from build123d import *

# Parameters (mm, degrees)
SALIENTE_EXTRUIR1_DEPTH = 3


with BuildPart() as part:
    # Croquis1 → Saliente-Extruir1 (new body)
    with BuildSketch(Plane.XY):
        with BuildLine():
            Line((77.13407836, 15), (-77.13407836, 15))
            add(Edge.make_bspline(
                [(-77.13407836, 15), (-77.871262638, 15), (-78.576496818, 14.787307583), (-79.282235227, 14.574463094), (-79.896125243, 14.167315569)],
                knots=[0, 0, 0, 0.5, 0.5, 1, 1, 1], degree=2))
            ThreePointArc((-79.896125243, 14.167315569), (-87.5, 0), (-79.896125243, -14.167315569))
            add(Edge.make_bspline(
                [(-79.896125243, -14.167315569), (-79.281776873, -14.574767086), (-78.576496886, -14.787307562), (-77.870712638, -15), (-77.13407836, -15)],
                knots=[0, 0, 0, 0.5, 0.5, 1, 1, 1], degree=2))
            Line((-77.13407836, -15), (77.13407836, -15))
            add(Edge.make_bspline(
                [(77.13407836, -15), (77.871262638, -15), (78.576496818, -14.787307583), (79.282235227, -14.574463094), (79.896125243, -14.167315569)],
                knots=[0, 0, 0, 0.5, 0.5, 1, 1, 1], degree=2))
            ThreePointArc((79.896125243, -14.167315569), (87.5, 0), (79.896125243, 14.167315569))
            add(Edge.make_bspline(
                [(79.896125243, 14.167315569), (79.281776873, 14.574767086), (78.576496886, 14.787307562), (77.870712638, 15), (77.13407836, 15)],
                knots=[0, 0, 0, 0.5, 0.5, 1, 1, 1], degree=2))
        make_face()
    extrude(amount=SALIENTE_EXTRUIR1_DEPTH)


solid = part.part
Design review of the part built by this model. Coordinates are the model's own, in mm. Give positions to 0.01 mm unless a question says otherwise; leave off trailing zeros. Order: outer loops, then holes, each group sorted by start corner. A loop starts at its lowest first (then second) coordinate and runs counter-clockwise, first axis right, second up.
1. Add section B-B, the plane y = -7.5. State the section outline as (x, z) points, then the cut area to 3 significant figures.
Solution:
outline: (-85.76, 0) - (85.76, 0) - (85.76, 3) - (-85.76, 3) - close
area: 515 mm2
2. For pin 1 Ø2 at (x, y) = (69.5, -6.5) entering from -Z, flat-tipped, find the tip position at first contact; note if it passes through.
Solution:
pin 1: stops at z = 0
3. Add section A-A, the plane y = 8. State the section outline as (x, z) points, then the cut area to 3 significant figures.
Solution:
outline: (-85.5, 0) - (85.5, 0) - (85.5, 3) - (-85.5, 3) - close
area: 513 mm2
4. To check wall thickness, follow L1, parallel to X at y = 6, z = 1.85; L2, parallel to X at y = 9, z = 2.2. State the ranges of each line that lie inside material, in increasing order.
Solution:
L1: x = -86.41 to 86.41
L2: x = -84.92 to 84.92
